Answer from the drawing. Dimensions are ordinates in mm from the lowest x, y and z of the part. A direction names the side the tool comes from. Coordinates: 2 decimals unless noted, no trailing zeros. Write each loop counter-clockwise with the first axis right and the second up, starting at its lowest first coordinate (ties: lowest second). Pieces come first, ordered by that corner, then holes.
1) Which of the six approach directions +Z, -Z, +X, -X, +Y, -Y give full straight-line access (tool end or side, diameter ignored) to the marked faces 1, 2 and 3?
2) The part is cut by section A-A (z = 11). Determine the outline of the cut face in (x, y).
3) The part is cut by section D-D (x = 7). Determine the outline of the cut face in (y, z), then the cut area to 3 significant figures.
4) The part is cut by section B-B (x = 27). Determine the outline of the cut face in (y, z), then the cut area to 3 significant figures.
5) Each of these flat-tipped pins is pushed along its axis until it touches: pin 1 Ø16 at (x, y) = (27, 33.5) entering from -Z; pin 2 Ø4 at (y, z) = (25, 15) entering from -X; pin 3 Ø5.5 at (x, z) = (35, 13.5) entering from -Y; pin 4 Ø1.5 at (x, y) = (5.5, 368.5) entering from -Z. Where does it stop, or does it pass through?
6) The part is cut by section C-C (y = 229). Determine the outline of the cut face in (x, z).
7) Find the intervals of material crossed by line 1 (X direction, y = 347.5, z = 12.75); line 2 (Y direction, x = 24, z = 1.5); line 3 (Z direction, x = 25, y = 441), in increasing order.
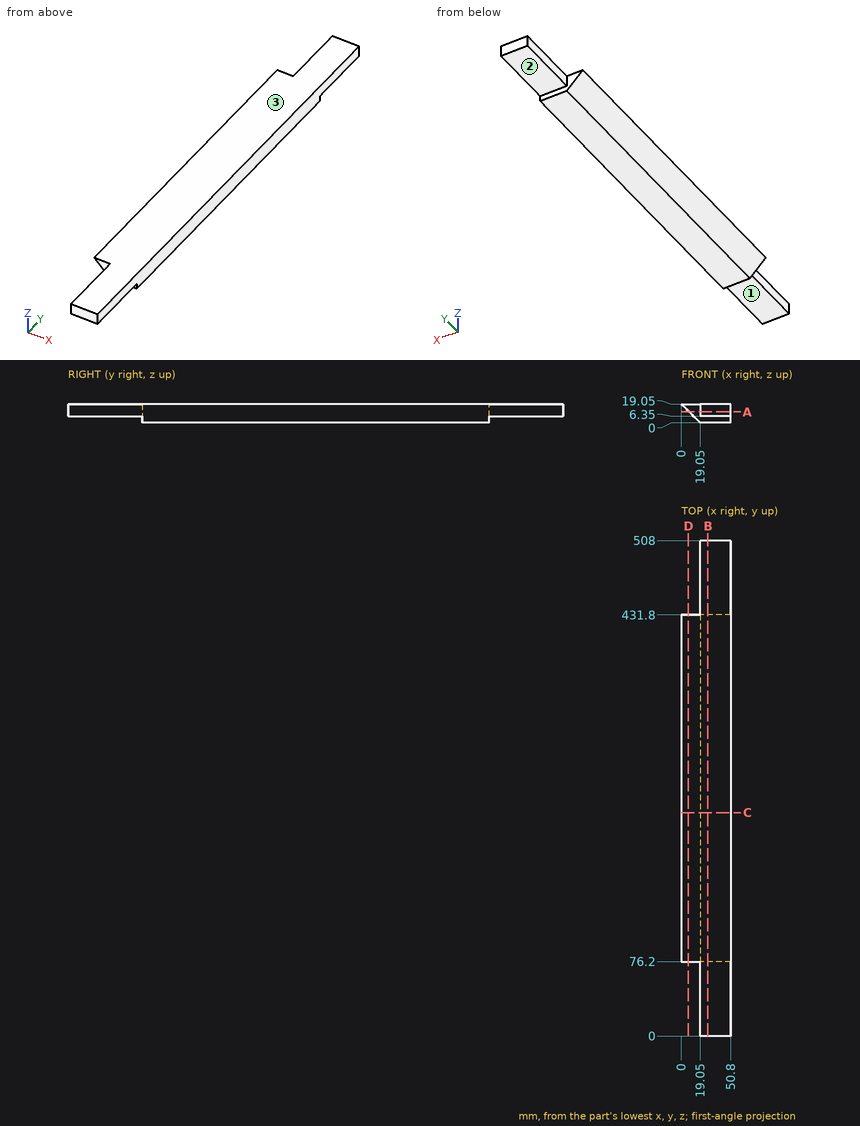
Reported:
1. face 1: -Z, +X, -X, -Y
1. face 2: -Z, +X, -X, +Y
1. face 3: +Z, +X, -X, +Y, -Y
2. outline: (8.05, 76.2) - (19.05, 76.2) - (19.05, 0) - (50.8, 0) - (50.8, 508) - (19.05, 508) - (19.05, 431.8) - (8.05, 431.8) - close
3. outline: (76.2, 12.05) - (431.8, 12.05) - (431.8, 19.05) - (76.2, 19.05) - close
3. area: 2,490 mm2
4. outline: (0, 6.35) - (76.2, 6.35) - (76.2, 0) - (431.8, 0) - (431.8, 6.35) - (508, 6.35) - (508, 19.05) - (0, 19.05) - close
4. area: 8,710 mm2
5. pin 1: stops at z = 6.35
5. pin 2: stops at x = 19.05
5. pin 3: stops at y = 0
5. pin 4: stops at z = 12.8
6. outline: (0, 19.05) - (19.05, 0) - (50.8, 0) - (50.8, 19.05) - close
7. line 1: x = 6.3 to 50.8
7. line 2: y = 76.2 to 431.8
7. line 3: z = 6.35 to 19.05
